Part model, mm, in its own coordinate system. Give positions to 0.01 mm unless a question says otherwise; leave off trailing zeros. Order: outer loops, then holes, each group sorted by start corner. A loop starts at its lowest first (then second) coordinate and runs counter-clockwise, first axis right, second up. Notation, with made-up numbers: M -34.75,-33.75 L -22.75,-33.75 A11 cw -22.75,-21.75 Z; hole C -39.75,62.25 d4. An arc over 180 degrees is marked long. One line per question, with ' | ' between items.
```python
from build123d import *

# Parameters (mm, degrees)
F0_W     = 42.3045453848
F0_H     = 2.0955
F1_DEPTH = 5.842
F0_H_2   = 2.9395276724
F2_DEPTH = 5.08


with BuildPart() as f1:
    # F0 (on Right) → F1 (new body)
    with BuildSketch(Plane.YZ):
        with BuildLine():
            Line((-27.856127011, -0.0136474585), (-27.856127011, 2.0818525415))
            ThreePointArc((-27.856127011, 2.0818525415), (-29.51683868, 1.7387763651), (-30.9056579084, 0.7657164176))
            Line((-30.9056579084, 0.7657164176), (-30.7041171732, 0.7142089649))
            Line((-30.7041171732, 0.7142089649), (-27.856127011, -0.0136474585))
        make_face()
        with Locations((-6.7038543186, 1.0341025415)):
            Rectangle(F0_W, F0_H)
        Polygon((19.4500260153, 2.0818525415), (14.4484183737, 2.0818525415), (14.4484183737, -0.0136474585), (19.953361936, 0.7142089649), (19.953361936, 2.0818525415), align=None)
    extrude(amount=F1_DEPTH)

    # F0 (on Right) → F2 (join)
    with BuildSketch(Plane.YZ):
        with BuildLine():
            Line((-27.856127011, -2.953175131), (-27.856127011, -0.0136474585))
            Line((-27.856127011, -0.0136474585), (-30.7041171732, 0.7142089649))
            ThreePointArc((-30.7041171732, 0.7142089649), (-30.1778049641, -1.816599044), (-27.856127011, -2.953175131))
        make_face()
        with Locations((-6.7038543186, -1.4834112948)):
            Rectangle(F0_W, F0_H_2)
        with BuildLine():
            Line((19.953361936, 0.7142089649), (14.4484183737, -0.0136474585))
            Line((14.4484183737, -0.0136474585), (14.4484183737, -2.953175131))
            Line((14.4484183737, -2.953175131), (16.2859778402, -2.953175131))
            ThreePointArc((16.2859778402, -2.953175131), (18.8792100035, -1.8790231985), (19.953361936, 0.7142089649))
        make_face()
    extrude(amount=F2_DEPTH)


solid = f1.part
```
1. Slice it at C-C on z = -0.6. Give the cut face in (x, y), then the cut area to 3 significant figures.
Worked out:
outline: M 0,-30.74 L 5.08,-30.74 L 5.08,19.71 L 0,19.71 Z | area: 256 mm2
2. Slice it at A-A on x = 3.9. Give the cut face in (y, z), then the cut area to 3 significant figures.
Worked out:
outline: M -30.91,0.77 L -30.7,0.71 A2.94 ccw -27.86,-2.95 L 16.29,-2.95 A3.67 ccw 19.95,0.71 L 19.95,2.08 L -27.86,2.08 A4.19 ccw Z | area: 250 mm2
3. Slice it at B-B on y = -10.5. Give the cut face in (x, z).
Worked out:
outline: M 0,-2.95 L 5.08,-2.95 L 5.08,-0.01 L 5.84,-0.01 L 5.84,2.08 L 0,2.08 Z
4. Probe L1, parallel to X at y = -27.5, z = -1.7; L2, parallel to Z at x = 1.65, y = 16.5; L3, parallel to Z at x = 5.35, y = 6. List the from-to ranges inside material, lowest first. Write a range as from..to.
Worked out:
L1: x = 0..5.08 | L2: z = -2.95..2.08 | L3: z = -0.01..2.08
5. Drop flat-ended pins along their axis: pin 1 (0.6 mm diameter, centred on x = 5.5, y = -4.5, fed in from -Z); pin 2 (1.5 mm diameter, centred on y = 1, z = -2, fed in from +X); pin 3 (1 mm diameter, centred on x = 3.5, z = -0.5, fed in from +Y). Give the stop position or say it passes through.
Worked out:
pin 1: stops at z = -0.01 | pin 2: stops at x = 5.08 | pin 3: stops at y = 19.88
